```python
from build123d import *

# Parameters (mm, degrees)
SKETCH1_W             = 125
SKETCH1_H             = 110
SKETCH1_R             = 2.75
BOSS_EXTRUDE1_DEPTH   = 10
M5_TAPPED_HOLE3_D     = 4.2
M5_TAPPED_HOLE3_DEPTH = 16
M5_TAPPED_HOLE3_TIP   = 1.2618073
M5_TAPPED_HOLE4_D     = 4.2
M5_TAPPED_HOLE4_DEPTH = 16
M5_TAPPED_HOLE4_TIP   = 1.2618073
SKETCH13_R            = 5
CUT_EXTRUDE1_DEPTH    = 5.7


with BuildPart() as part:
    # Sketch1 → Boss-Extrude1 (new body)
    with BuildSketch(Plane(origin=(0, 0, 0), x_dir=(1, 0, 0), z_dir=(0, 1, 0))):
        Rectangle(SKETCH1_W, SKETCH1_H)
        with Locations((7.5, -11)):
            Circle(SKETCH1_R, mode=Mode.SUBTRACT)
        with Locations((-7.5, -47)):
            Circle(SKETCH1_R, mode=Mode.SUBTRACT)
    extrude(amount=BOSS_EXTRUDE1_DEPTH)

    # M5 Tapped Hole3
    with Locations(Plane(origin=(0, 0, -55), x_dir=(-1, 0, 0), z_dir=(0, 0, -1))):
        with Locations((-47.5, 5), (47.5, 5)):
            Hole(M5_TAPPED_HOLE3_D / 2, depth=M5_TAPPED_HOLE3_DEPTH)
            with Locations((0, 0, -(M5_TAPPED_HOLE3_DEPTH + M5_TAPPED_HOLE3_TIP / 2))):  # 118° drill point
                Cone(0, M5_TAPPED_HOLE3_D / 2, M5_TAPPED_HOLE3_TIP, mode=Mode.SUBTRACT)

    # M5 Tapped Hole4
    with Locations(Plane.XY.offset(55)):
        with Locations((-47.5, 5), (47.5, 5)):
            Hole(M5_TAPPED_HOLE4_D / 2, depth=M5_TAPPED_HOLE4_DEPTH)
            with Locations((0, 0, -(M5_TAPPED_HOLE4_DEPTH + M5_TAPPED_HOLE4_TIP / 2))):  # 118° drill point
                Cone(0, M5_TAPPED_HOLE4_D / 2, M5_TAPPED_HOLE4_TIP, mode=Mode.SUBTRACT)

    # Sketch13 → Cut-Extrude1 (cut)
    with BuildSketch(Plane(origin=(0, 0, 0), x_dir=(-1, 0, 0), z_dir=(0, -1, 0))):
        with Locations((-7.5, -11)):
            Circle(SKETCH13_R)
        with Locations((7.5, -47)):
            Circle(SKETCH13_R)
    extrude(amount=-CUT_EXTRUDE1_DEPTH, mode=Mode.SUBTRACT)


solid = part.part
```
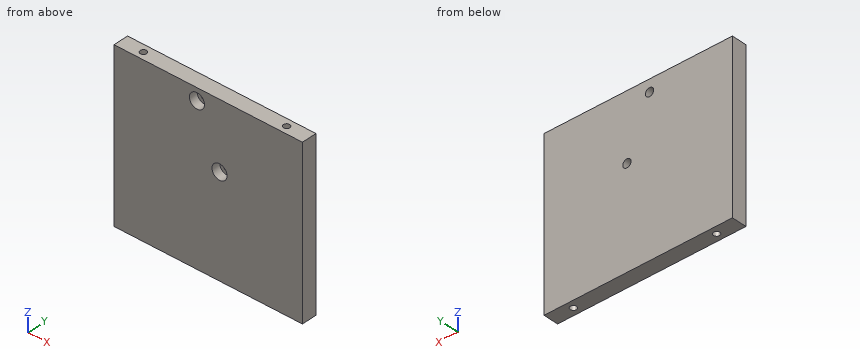
Part model, mm, in its own coordinate system. Coordinates: 2 decimals unless noted, no trailing zeros. Write each loop counter-clockwise with the first axis right and the second up, starting at its lowest first coordinate (ties: lowest second). Pieces come first, ordered by that corner, then holes.
Item 1: Slice it at C-C (z = 11). Write the cut outline in (x, y).
Item 2: Pin check, flat tips, straight feed: pin 1 (6 mm diameter, centred on x = -7.5, z = 47, fed in from -Y); pin 2 (2.5 mm diameter, centred on x = 47.5, y = 5, fed in from +Z); pin 3 (4 mm diameter, centred on x = -47.5, y = 5, fed in from +Z). Stop position of each tip, or through.
Item 3: Slice it at B-B (x = 7.5). Write the cut outline in (y, z).
Item 4: Probe line 1 (X direction, y = 5, z = -42); line 2 (Y direction, x = 47.5, z = 47.75); line 3 (Z direction, x = 7.5, y = 3.9). List the from-to ranges inside material, lowest first.
Item 5: Slice it at A-A (z = 47). Write the cut outline in (x, y).
Item 6: Slice it at D-D (z = -44.5). Write the cut outline in (x, y).
Results found:
1. outline: (-62.5, 0) - (2.5, 0) - (2.5, 5.7) - (4.75, 5.7) - (4.75, 10) - (-62.5, 10) - close; (10.25, 5.7) - (12.5, 5.7) - (12.5, 0) - (62.5, 0) - (62.5, 10) - (10.25, 10) - close
2. pin 1: stops at y = 5.7
2. pin 2: stops at z = 38.49
2. pin 3: stops at z = 38.94
3. outline: (0, -55) - (10, -55) - (10, 8.25) - (5.7, 8.25) - (5.7, 6) - (0, 6) - close; (0, 16) - (5.7, 16) - (5.7, 13.75) - (10, 13.75) - (10, 55) - (0, 55) - close
4. line 1: x = -62.5 to -49.6, -45.4 to 45.4, 49.6 to 62.5
4. line 2: y = 0 to 2.9, 7.1 to 10
4. line 3: z = -55 to 6, 16 to 55
5. outline: (-62.5, 0) - (-12.5, 0) - (-12.5, 5.7) - (-10.25, 5.7) - (-10.25, 10) - (-62.5, 10) - close; (-4.75, 5.7) - (-2.5, 5.7) - (-2.5, 0) - (62.5, 0) - (62.5, 10) - (-4.75, 10) - close; hole circle Ø4.2 at (-47.5, 5); hole circle Ø4.2 at (47.5, 5)
6. outline: (-62.5, 0) - (62.5, 0) - (62.5, 10) - (-62.5, 10) - close; hole circle Ø4.2 at (-47.5, 5); hole circle Ø4.2 at (47.5, 5)
